Autodesk Inventor part; units mm, degrees
ref_plane "YZ Plane" through (0, 0, 0) normal (1, 0, 0) x (0, 1, 0)
ref_plane "XZ Plane" through (0, 0, 0) normal (0, 1, 0) x (-1, 0, 0)
ref_plane "XY Plane" through (0, 0, 0) normal (0, 0, 1) x (1, 0, 0)
sketch "Sketch1" plane through (0, 0, 0) normal (0, 0, 1) x (1, 0, 0)
  line L0 (0, 0) -> (76.2, 0)
  line L1 (76.2, 0) -> (76.2, 50.8)
  line L2 (0, 50.8) -> (0, 0)
  line L3 (25.4, 152.4) -> (0, 152.4)
  line L4 (0, 152.4) -> (0, 50.8)
  line L5 (25.4, 152.4) -> (76.2, 50.8)
  circle A0 centre (12.7, 12.7) radius 3.2512
  circle A1 centre (12.7, 38.1) radius 3.2512
  circle A2 centre (12.7, 63.5) radius 3.2512
  circle A3 centre (12.7, 88.9) radius 3.2512
  circle A4 centre (12.7, 114.3) radius 3.2512
  circle A5 centre (12.7, 139.7) radius 3.2512
  circle A6 centre (38.1, 12.7) radius 3.2512
  circle A7 centre (63.5, 12.7) radius 3.2512
  circle A8 centre (12.7, 38.1) radius 3.2512
  circle A9 centre (38.1, 38.1) radius 3.2512
  circle A10 centre (63.5, 38.1) radius 3.2512
  dimension "d4" = 101.6
  dimension "d5" = 50.8
  dimension "d6" = 25.4
  dimension "d7" = 50.8
  dimension "d8" = 101.6
  dimension "d9" = 50.8
  dimension "d10" = 76.2
  dimension "d11" = 6.5024
  dimension "d12" = 12.7
  dimension "d13" = 12.7
  dimension "d16" = 25.4
  dimension "d23" = 25.4
  dimension "d26" = 25.4
extrude "Extrusion1" add sketch "Sketch1" along normal blind 6.35
properties part number "6x3"
Work out the finished part from the listing and answer in its coordinate system (mm). Give positions to 0.01 mm unless a question says otherwise; leave off trailing zeros. Loops run counter-clockwise (first coordinate to the right, second up) from the corner with the lowest first, then second, coordinate; pieces in that order, holes last. Notation, with made-up numbers: (-17.5, -23.75) -> (19.5, -23.75) arc R10 ccw to (19.5, -17.75) -> close; hole circle Ø1 at (76.5, 74.25). An arc over 180 degrees is marked (long way). Write item = value, one per line. Start each with the question number.
(1) Find section D-D on y = 12.7. Give the vertices of the cut face in (x, z).
(2) Find section C-C on x = 12.7. Give the vertices of the cut face in (y, z).
(3) Find section B-B on y = 88.9. Give the vertices of the cut face in (x, z), and give its area (3 significant figures).
(4) The mould has two halves that part along X. Classify faces 1 (the flat face through (29, 60, 0)), 2 (the cylindrical face through (14.2, 66.384, 3.131)), 3 (the flat face through (50.444, 102.311, 3.131)): +X half, -X half, draft (parallel to the pull), parting line (faces both ways), or undercut.
(5) Given pin 1 Ø6 at (x, y) = (12.7, 139.7) entering from -Z; pin 2 Ø2 at (x, z) = (56.5, 2.5) entering from +Y, each flat-ended and moving along its own axis, determine where each tip first touches the part or whether it passes through.
(6) Find section A-A on x = 63.5. Give the vertices of the cut face in (y, z).
(7) Find the intervals of material crossed by probe 1 along Y at (x, z) = (63.5, 2.75); probe 2 along X at (y, z) = (10, 5); probe 3 along X at (y, z) = (38, 1.25), in increasing order. Write a range as from..to.
From the geometry:
q1.outline = (0, 0) -> (9.45, 0) -> (9.45, 6.35) -> (0, 6.35) -> close; (15.95, 0) -> (34.85, 0) -> (34.85, 6.35) -> (15.95, 6.35) -> close; (41.35, 0) -> (60.25, 0) -> (60.25, 6.35) -> (41.35, 6.35) -> close; (66.75, 0) -> (76.2, 0) -> (76.2, 6.35) -> (66.75, 6.35) -> close
q2.outline = (0, 0) -> (9.45, 0) -> (9.45, 6.35) -> (0, 6.35) -> close; (15.95, 0) -> (34.85, 0) -> (34.85, 6.35) -> (15.95, 6.35) -> close; (41.35, 0) -> (60.25, 0) -> (60.25, 6.35) -> (41.35, 6.35) -> close; (66.75, 0) -> (85.65, 0) -> (85.65, 6.35) -> (66.75, 6.35) -> close; (92.15, 0) -> (111.05, 0) -> (111.05, 6.35) -> (92.15, 6.35) -> close; (117.55, 0) -> (136.45, 0) -> (136.45, 6.35) -> (117.55, 6.35) -> close; (142.95, 0) -> (152.4, 0) -> (152.4, 6.35) -> (142.95, 6.35) -> close
q3.outline = (0, 0) -> (9.45, 0) -> (9.45, 6.35) -> (0, 6.35) -> close; (15.95, 0) -> (57.15, 0) -> (57.15, 6.35) -> (15.95, 6.35) -> close
q3.area = 322 mm^2
q4.face_1 = draft
q4.face_2 = undercut
q4.face_3 = +X half
q5.pin_1 = through
q5.pin_2 = 92.2
q6.outline = (0, 0) -> (9.45, 0) -> (9.45, 6.35) -> (0, 6.35) -> close; (15.95, 0) -> (34.85, 0) -> (34.85, 6.35) -> (15.95, 6.35) -> close; (41.35, 0) -> (76.2, 0) -> (76.2, 6.35) -> (41.35, 6.35) -> close
q7.probe_1 = 0..9.45, 15.95..34.85, 41.35..76.2
q7.probe_2 = 0..10.89, 14.51..36.29, 39.91..61.69, 65.31..76.2
q7.probe_3 = 0..9.45, 15.95..34.85, 41.35..60.25, 66.75..76.2
